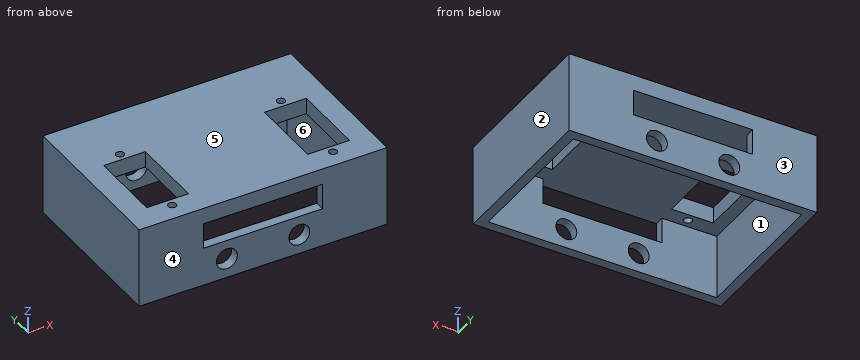
Autodesk Inventor part; units mm, degrees
ref_plane "YZ Plane" through (0, 0, 0) normal (1, 0, 0) x (0, 1, 0)
ref_plane "XZ Plane" through (0, 0, 0) normal (0, 1, 0) x (-1, 0, 0)
ref_plane "XY Plane" through (0, 0, 0) normal (0, 0, 1) x (1, 0, 0)
sketch "Sketch1" plane through (0, 0, 0) normal (0, 0, 1) x (1, 0, 0)
  line L0 (0, 0) -> (-77, 0)
  line L1 (-77, 0) -> (-77, -51.3)
  line L2 (-77, -51.3) -> (0, -51.3)
  line L3 (0, -51.3) -> (0, 0)
  line L4 (-7, -20.3) -> (-20, -20.3)
  line L5 (-20, -20.3) -> (-20, -43.3)
  line L6 (-20, -43.3) -> (-7, -43.3)
  line L7 (-7, -43.3) -> (-7, -20.3)
  line L8 (-57, -20.3) -> (-70, -20.3)
  line L9 (-70, -20.3) -> (-70, -43.3)
  line L10 (-70, -43.3) -> (-57, -43.3)
  line L11 (-57, -43.3) -> (-57, -20.3)
  point P0 (-7, -31.8)
  point P1 (0, -25.65)
  point P2 (-13.5, -20.3)
  point P3 (-63.5, -20.3)
  dimension "d1" = 51.3
  dimension "d4" = 23
  dimension "d5" = 13
  dimension "d7" = 7
  dimension "d18" = 50
  dimension "d19" = 7
  dimension "d20" = 8
extrude "Extrusion1" add sketch "Sketch1" along normal blind 5
sketch "Sketch3" plane through (0, 0, 5) normal (0, 0, 1) x (1, 0, 0)
  line L0 (-77, 0) -> (-77, -51.3)
  line L1 (-77, -51.3) -> (0, -51.3)
  line L2 (0, -51.3) -> (0, 0)
  line L3 (0, 0) -> (-77, 0)
  line L4 (-7, -20.3) -> (-7, -43.3)
  line L5 (-7, -43.3) -> (-20, -43.3)
  line L6 (-20, -43.3) -> (-20, -20.3)
  line L7 (-20, -20.3) -> (-7, -20.3)
  line L8 (-20, -20.3) -> (-7, -20.3)
  line L9 (-70, -20.3) -> (-57, -20.3)
  point P0 (-13.5, -17.9)
  point P1 (-13.5, -45.7)
  point P2 (-13.5, -20.3)
  point P3 (-13.5, -20.3)
  point P4 (-13.5, -43.3)
  point P5 (-63.5, -17.9)
  point P6 (-63.5, -45.7)
  point P7 (-63.5, -20.3)
  point P8 (-63.5, -20.3)
  dimension "d8" = 27.8
  dimension "d9" = 2.4
  dimension "d10" = 2.4
hole "Hole1" at (-13.5, -17.9, 5) at (-13.5, -45.7, 5) at (-63.5, -45.7, 5) at (-63.5, -17.9, 5) direction (0, 0, -1) diameter 2.5 end through all
sketch "Sketch4" plane through (-77, 0, 0) normal (0, 1, 0) x (1, 0, 0)
  line L0 (77, 0) -> (0, 0)
  line L1 (0, 0) -> (0, -5)
  line L2 (77, -5) -> (0, -5)
  line L3 (77, 0) -> (77, -5)
  line L4 (77, 20) -> (0, 20)
  line L5 (0, 20) -> (0, 8)
  line L6 (0, 8) -> (77, 8)
  line L7 (77, 8) -> (77, 20)
  line L8 (0, 0) -> (77, 0)
  line L9 (77, 8) -> (57, 8)
  line L10 (57, 8) -> (57, 0)
  line L11 (57, 0) -> (77, 0)
  line L12 (77, 0) -> (77, 8)
  line L13 (0, 0) -> (20, 0)
  line L14 (20, 0) -> (20, 8)
  line L15 (20, 8) -> (0, 8)
  line L16 (0, 8) -> (0, 0)
  circle A0 centre (27.25, 13.95) radius 3.25
  point P0 (77, 4)
  point P1 (57, 8)
  dimension "d21" = 12
  dimension "d22" = 8
  dimension "d23" = 20
  dimension "d24" = 20
  dimension "d41" = 5.95
extrude "Extrusion2" add sketch "Sketch4" against normal blind 3 contours L0 L10 L6 L12 | L6 L5 L4 L7 | L0 L16 L6 L14 | A0
extrude "Extrusion3" add sketch "Sketch4" along normal blind 3 from surface at -51.3 contours L0 L10 L6 L12 | L6 L5 L4 L7 | L0 L16 L6 L14 | A0
sketch "Sketch5" plane through (0, 0, 0) normal (0, 0, -1) x (-1, 0, 0)
  line L0 (0, 0) -> (77, 0)
  line L1 (0, 0) -> (0, -3)
  line L2 (77, -3) -> (0, -3)
  line L3 (77, 0) -> (77, -3)
  line L4 (20, 0) -> (20, -3)
  line L5 (57, 0) -> (57, -3)
  line L6 (0, -48.3) -> (77, -48.3)
  line L7 (20, -3) -> (0, -3)
  line L8 (0, -3) -> (0, -48.3)
  line L9 (0, -48.3) -> (20, -48.3)
  line L10 (20, -48.3) -> (20, -3)
  line L11 (20, -3) -> (57, -3)
  line L12 (57, -3) -> (77, -3)
  line L13 (77, -3) -> (77, -48.3)
  line L14 (77, -48.3) -> (57, -48.3)
  line L15 (57, -48.3) -> (57, -3)
  line L16 (0, -3) -> (3, -3)
  line L17 (3, -3) -> (3, -48.3)
  line L18 (3, -48.3) -> (0, -48.3)
  line L19 (0, -48.3) -> (0, -3)
  line L20 (77, -3) -> (74, -3)
  line L21 (74, -3) -> (74, -48.3)
  line L22 (74, -48.3) -> (77, -48.3)
  line L23 (77, -48.3) -> (77, -3)
  point P0 (0, -3)
  point P1 (20, -48.3)
  point P2 (3, -48.3)
  dimension "d42" = 3
  dimension "d43" = 3
extrude "Extrusion4" add sketch "Sketch5" along normal up to surface (20 mm away) contours L2 L17 L6 L8 | L13 L6 L21 L2
sketch "Sketch6" plane through (-77, 0, 5) normal (0, 1, 0) x (1, 0, 0)
  line L0 (20, 5) -> (20, 13)
  line L1 (20, 13) -> (57, 13)
  line L2 (57, 13) -> (57, 5)
  line L3 (57, 5) -> (20, 5)
  line L4 (0, 25) -> (0, 0)
  line L5 (77, 0) -> (0, 0)
  line L6 (77, 25) -> (77, 0)
  line L7 (77, 25) -> (0, 25)
  point P0 (77, 5)
  point P1 (49.75, 18.95)
  point P2 (27.25, 18.95)
  dimension "d31" = 27.25
  dimension "d32" = 27.25
  dimension "d33" = 6.05
hole "Hole2" at (-27.25, 0, -13.95) at (-49.75, 0, -13.95) direction (0, -1, 0) diameter 6.5 end through all
equation "\"d19\" = d7"
equation "\"d23\" = d24"
equation "\"d43\" = d42"
properties part number "Test Frame_3DPrint"
Here's how the part is built. I have some questions about the finished solid (model axes, mm). Face numbers are marked on the shaded views. A direction names the side the tool comes from. Round coordinates to 2 decimals unless told otherwise and drop trailing zeros. Loops run counter-clockwise (first coordinate to the right, second up) from the corner with the lowest first, then second, coordinate; pieces in that order, holes last.
1. We'd pull the mould along Y, two halves only. Please class the marked faces 1, 2, 3 and 4: +Y half, -Y half, draft (parallel to the pull), parting line (faces both ways), or undercut.
Answer list:
face 1: undercut
face 2: draft
face 3: +Y half
face 4: -Y half
2. For P1, Ø15.5, axis at x = -37.5, y = -20.5, coming from the -Z side; P2, Ø1.5, axis at x = -63.5, y = -17.9, coming from the +Z side, each with a flat end and sliding along its axis, tell me the tip position at first contact or that it passes through.
Answer list:
P1: stops at z = 0
P2: passes through
3. Which directions (+Z, -Z, +X, -X, +Y, -Y) give clear straight access to the entire face, cutting with the end or side of a thin tool? Please do the marked faces 5 and 6.
Answer list:
face 5: +Z, +X, -X, +Y, -Y
face 6: -Z
4. If we section it at A-A on y = -45.7: Write out the boundary of the cut face in (x, z), plus the area to 3 significant figures.
Answer list:
outline: (-77, -20) - (-74, -20) - (-74, 0) - (-64.75, 0) - (-64.75, 5) - (-77, 5) - close; (-62.25, 0) - (-14.75, 0) - (-14.75, 5) - (-62.25, 5) - close; (-12.25, 0) - (-3, 0) - (-3, -20) - (0, -20) - (0, 5) - (-12.25, 5) - close
area: 480 mm2
5. If we section it at D-D on x = -13.5: Write out the boundary of the cut face in (y, z), plus the area to 4 significant figures.
Answer list:
outline: (-51.3, -20) - (-48.3, -20) - (-48.3, 0) - (-46.95, 0) - (-46.95, 5) - (-51.3, 5) - close; (-44.45, 0) - (-43.3, 0) - (-43.3, 5) - (-44.45, 5) - close; (-20.3, 0) - (-19.15, 0) - (-19.15, 5) - (-20.3, 5) - close; (-16.65, 0) - (-3, 0) - (-3, -20) - (0, -20) - (0, 5) - (-16.65, 5) - close
area: 236.5 mm2
6. If we section it at C-C on z = -13.95: Write out the boundary of the cut face in (x, y).
Answer list:
outline: (-77, -51.3) - (-53, -51.3) - (-53, -48.3) - (-74, -48.3) - (-74, -3) - (-53, -3) - (-53, 0) - (-77, 0) - close; (-46.5, -51.3) - (-30.5, -51.3) - (-30.5, -48.3) - (-46.5, -48.3) - close; (-46.5, -3) - (-30.5, -3) - (-30.5, 0) - (-46.5, 0) - close; (-24, -51.3) - (0, -51.3) - (0, 0) - (-24, 0) - (-24, -3) - (-3, -3) - (-3, -48.3) - (-24, -48.3) - close
7. If I drill on line 1 along X through (y, z) = (-1.2, -13.95); line 2 along X through (y, z) = (-20.5, 1.5); line 3 along Z through (x, y) = (-27, -49), over which ranges is the centre line in solid material (lowest first)?
Answer list:
line 1: x = -77 to -53, -46.5 to -30.5, -24 to 0
line 2: x = -77 to -70, -57 to -20, -7 to 0
line 3: z = -20 to -17.19, -10.71 to -8, 0 to 5
8. If we section it at B-B on x = -27.25: Write out the boundary of the cut face in (y, z), plus the area to 4 significant figures.
Answer list:
outline: (-51.3, -20) - (-48.3, -20) - (-48.3, -17.2) - (-51.3, -17.2) - close; (-51.3, -10.7) - (-48.3, -10.7) - (-48.3, -8) - (-51.3, -8) - close; (-51.3, 0) - (0, 0) - (0, 5) - (-51.3, 5) - close; (-3, -20) - (0, -20) - (0, -17.2) - (-3, -17.2) - close; (-3, -10.7) - (0, -10.7) - (0, -8) - (-3, -8) - close
area: 289.5 mm2
